Geometry check sheet. Reference: the model listing, model coordinates, mm. A direction names the side the tool comes from. Round coordinates to 2 decimals unless told otherwise and drop trailing zeros. Order: outer loops, then holes, each group sorted by start corner. A loop starts at its lowest first (then second) coordinate and runs counter-clockwise, first axis right, second up.
(1) Go/stop test with flat-tipped pins: pin 1 (1 mm diameter, centred on y = 5, z = 6, fed in from -X); pin 2 (1 mm diameter, centred on x = -3.5, z = 1, fed in from -Y); pin 3 (1.6 mm diameter, centred on x = 4, z = 31, fed in from +Y). Record where each tip stops, or that it passes through.
(2) Set-up check for faces 5 (the face through (4, 7.262, 1)), 6 (the face through (-4, 6.185, 31)), 7 (the face through (-7, 10.401, 1)), 8 (the face through (2.085, 7, 31)): record each of +Z, -Z, +X, -X, +Y, -Y from which the full face is reachable in a straight line by a thin tool's end or side.
(3) Release check for a two-part mould opening along X. For faces 1 (the face through (4, 6.185, 31)), 2 (the face through (-2.085, 7, 1)), 3 (the face through (8.41, 11, 31)), 4 (the face through (-5.247, 7, 1)) record: +X half, -X half, draft (parallel to the pull), parting line (faces both ways), or undercut.
(4) Material ranges on line 1 along Z through (x, y) = (-8.5, 4.5); line 2 along Y through (x, z) = (6, 21); line 3 along X through (y, z) = (9.5, 15.5), recorded low to high.
(5) Sectioned sample at C-C (x = 8). Record the boundary of the cut face in (y, z).
(6) Sectioned sample at D-D (z = 17). Record the boundary of the cut face in (x, y), plus the area to 3 significant figures.
(7) Sectioned sample at A-A (z = 30.5). Record the boundary of the cut face in (x, y), plus the area to 3 significant figures.
(8) Sectioned sample at B-B (y = 8.75). Record the boundary of the cut face in (x, z).
from build123d import *

# Parameters (mm, degrees)
EXTRUDE1_START      = 2
EXTRUDE1_DEPTH      = 28
EXTRUDE2_DEPTH      = 2
EXTRUDE2_DEPTH_BACK = 30
SKETCH4_W           = 3.162406988
SKETCH4_H           = 1.077560899
SKETCH4_H_2         = 1.0775609


with BuildPart() as part:
    # Sketch1 → Extrude1 (new body)
    with BuildSketch(Plane.XY.offset(EXTRUDE1_START)):
        with BuildLine():
            Line((5.75, 14.5), (-5.75, 14.5))
            ThreePointArc((-5.75, 14.5), (-11.5, 8.75), (-5.75, 3))
            Line((-5.75, 3), (5.75, 3))
            ThreePointArc((5.75, 3), (11.5, 8.75), (5.75, 14.5))
        make_face()
    extrude(amount=EXTRUDE1_DEPTH)

    # Sketch4 → Extrude2 (add, two sides: drawn at the far end of the back side and taken through both)
    with BuildSketch(Plane(origin=(0, 0, 2), x_dir=(-1, 0, 0), z_dir=(0, 0, -1)).offset(-EXTRUDE2_DEPTH_BACK)):
        with Locations((-6.82845657, 10.940259655)):
            Rectangle(SKETCH4_W, SKETCH4_H)
        with Locations((-3.666049582, 6.723717004)):
            Rectangle(SKETCH4_W, SKETCH4_H_2)
        with Locations((3.666049582, 6.723717004)):
            Rectangle(SKETCH4_W, SKETCH4_H_2)
        with Locations((6.82845657, 10.940259655)):
            Rectangle(SKETCH4_W, SKETCH4_H)
    extrude(amount=EXTRUDE2_DEPTH + EXTRUDE2_DEPTH_BACK)


solid = part.part
Answer below:
1. pin 1: stops at x = -10.49
1. pin 2: stops at y = 6.18
1. pin 3: stops at y = 7.26
2. face 5: -Z, +X, -X, +Y
2. face 6: +Z, +X, -X, -Y
2. face 7: -Z, +X, -X, -Y
2. face 8: +Z, +Y, -Y
3. face 1: draft
3. face 2: undercut
3. face 3: +X half
3. face 4: -X half
4. line 1: z = 2 to 30
4. line 2: y = 3.01 to 14.49
4. line 3: x = -11.45 to 11.45
5. outline: (3.46, 2) - (10.4, 2) - (10.4, 0) - (11.48, 0) - (11.48, 2) - (14.04, 2) - (14.04, 30) - (11.48, 30) - (11.48, 32) - (10.4, 32) - (10.4, 30) - (3.46, 30) - close
6. outline: (-5.75, 3) - (5.75, 3) arc R5.75 ccw to (5.75, 14.5) - (-5.75, 14.5) arc R5.75 ccw to start
6. area: 236 mm2
7. outline: (-8.41, 10.4) - (-5.25, 10.4) - (-5.25, 11.48) - (-8.41, 11.48) - close; (-5.25, 6.18) - (-2.08, 6.18) - (-2.08, 7.26) - (-5.25, 7.26) - close; (2.08, 6.18) - (5.25, 6.18) - (5.25, 7.26) - (2.08, 7.26) - close; (5.25, 10.4) - (8.41, 10.4) - (8.41, 11.48) - (5.25, 11.48) - close
7. area: 13.6 mm2
8. outline: (-11.5, 2) - (11.5, 2) - (11.5, 30) - (-11.5, 30) - close
